Check sheet for the modelled part. Datum: model origin and axes. Units: mm. A direction names the side the tool comes from. Coordinates: 2 decimals unless noted, no trailing zeros. Loops run counter-clockwise (first coordinate to the right, second up) from the corner with the lowest first, then second, coordinate; pieces in that order, holes last.
```python
from build123d import *

# Parameters (mm, degrees)
F2_R     = 1.2
F3_DEPTH = 4.5
F4_R     = 0.75
F5_DEPTH = 7
F6_R     = 0.75
F7_DEPTH = 25
F9_DEPTH = 25


with BuildPart() as f1:
    # F0 (on Front) → F1 (revolve)
    with BuildSketch(Plane.XZ):
        with BuildLine():
            ThreePointArc((-16.2961422592, -2.25), (-18.5461422592, 0), (-16.2961422592, 2.25))
            Line((-16.2961422592, 2.25), (-19.7961422592, 2.25))
            Line((-19.7961422592, 2.25), (-19.7961422592, -2.25))
            Line((-19.7961422592, -2.25), (-16.2961422592, -2.25))
        make_face()
        with BuildLine():
            Line((-16.2961422592, 1.75), (-16.2961422592, 2.25))
            ThreePointArc((-16.2961422592, 2.25), (-18.5461422592, 0), (-16.2961422592, -2.25))
            Line((-16.2961422592, -2.25), (-16.2961422592, -1.75))
            ThreePointArc((-16.2961422592, -1.75), (-18.0461422592, 0), (-16.2961422592, 1.75))
        make_face()
    revolve(axis=Axis((-4.3961422592, 0, -0.5702087656), (0, 0, -1)))

    # F2 (on face) → F3 (join)
    with BuildSketch(Plane.XY.offset(2.25)):
        with BuildLine():
            ThreePointArc((-18.1132848188, -7), (-19.7961422592, 0), (-18.1132848188, 7))
            Line((-18.1132848188, 7), (-28.8961422592, 7))
            Line((-28.8961422592, 7), (-28.8961422592, -7))
            Line((-28.8961422592, -7), (-18.1132848188, -7))
        make_face()
        with Locations((-24.3961422592, 0)):
            Circle(F2_R, mode=Mode.SUBTRACT)
        with BuildLine():
            Line((16.3026824594, 4.5), (10.3317224876, 4.5))
            ThreePointArc((10.3317224876, 4.5), (10.8348970536, 2.2749596589), (11.0038577408, 0))
            ThreePointArc((11.0038577408, 0), (10.8348970536, -2.2749596589), (10.3317224876, -4.5))
            Line((10.3317224876, -4.5), (16.3026824594, -4.5))
            Line((16.3026824594, -4.5), (16.3026824594, 4.5))
        make_face()
    extrude(amount=-F3_DEPTH)

    # F4 (on face) → F5 (cut)
    with BuildSketch(Plane(origin=(0, 7, 0), x_dir=(-1, 0, 0), z_dir=(0, 1, 0))):
        with Locations((24.3961422592, 0)):
            Circle(F4_R)
    extrude(amount=-F5_DEPTH, mode=Mode.SUBTRACT)

    # F6 (on face) → F7 (cut)
    with BuildSketch(Plane(origin=(0, 4.5, 0), x_dir=(-1, 0, 0), z_dir=(0, 1, 0))):
        with Locations((-13.5026824594, 0)):
            Circle(F6_R)
    extrude(amount=-F7_DEPTH, mode=Mode.SUBTRACT)

    # F8 (on face) → F9 (cut)
    with BuildSketch(Plane.XY.offset(2.25)):
        with BuildLine():
            ThreePointArc((7.5038577408, 0), (7.50007322, 0.3000954384), (7.4887220648, 0.6))
            Line((7.4887220648, 0.6), (5.0247731139, 0.6))
            Line((5.0247731139, 0.6), (5.0247731139, -0.6))
            Line((5.0247731139, -0.6), (7.4887220648, -0.6))
            ThreePointArc((7.4887220648, -0.6), (7.50007322, -0.3000954384), (7.5038577408, 0))
        make_face()
        with BuildLine():
            Line((16.3026824594, -0.6), (16.3026824594, 0.6))
            Line((16.3026824594, 0.6), (7.4887220648, 0.6))
            ThreePointArc((7.4887220648, 0.6), (7.50007322, 0.3000954384), (7.5038577408, 0))
            ThreePointArc((7.5038577408, 0), (7.50007322, -0.3000954384), (7.4887220648, -0.6))
            Line((7.4887220648, -0.6), (16.3026824594, -0.6))
        make_face()
    extrude(amount=-F9_DEPTH, mode=Mode.SUBTRACT)


solid = f1.part
```
1) Mould release check, pull along Z, two halves, no side actions. Record for faces 4 (the cylindrical face through (14.252, 2.577, 0.033)), 5 (the cylindrical face through (-3.3, 15.36, -0.03)), 6 (the flat face through (-16.4, -1.1, -2.25)): +Z half, -Z half, draft (parallel to the pull), parting line (faces both ways), or undercut.
Answer sheet:
face 4: undercut
face 5: draft
face 6: -Z half
2) Section check A-A on z = 0. Enter the section's corners in (x, y).
Answer sheet:
outline: (-28.9, -7) - (-18.11, -7) arc R15.4 ccw to (10.33, -4.5) - (12.75, -4.5) - (12.75, -0.6) - (9.24, -0.6) arc R13.65 cw (long way) to (9.24, 0.6) - (12.75, 0.6) - (12.75, 4.5) - (10.33, 4.5) arc R15.4 ccw to (-18.11, 7) - (-23.65, 7) - (-23.65, 0.94) arc R1.2 cw (long way) to (-25.15, 0.94) - (-25.15, 7) - (-28.9, 7) - close; (14.25, -4.5) - (16.3, -4.5) - (16.3, -0.6) - (14.25, -0.6) - close; (14.25, 0.6) - (16.3, 0.6) - (16.3, 4.5) - (14.25, 4.5) - close
3) Scan lines: line 1 (Y direction, x = 13.5, z = 1.1); line 2 (X direction, y = -4, z = -0.9); line 3 (X direction, y = 5.5, z = 0.1). Record each from-to range of solid material in increasing order.
Answer sheet:
line 1: y = -4.5 to -0.6, 0.6 to 4.5
line 2: x = -28.9 to -17.19, 8.39 to 16.3
line 3: x = -28.9 to -25.14, -23.65 to -16.89, 8.09 to 9.99
4) Set-up check for faces 1 (the flat face through (13, 4.5, 1)), 2 (the flat face through (12, 0.6, 0)), 3 (the flat face through (-23, 7, 0)): record each of +Z, -Z, +X, -X, +Y, -Y from which the full face is reachable in a straight line by a thin tool's end or side.
Answer sheet:
face 1: +Z, -Z, +X, +Y
face 2: +Z, -Z, +X
face 3: +Z, -Z, -X, +Y
5) Depth check by flat-ended pin: pin 1 (14.5 mm diameter, centred on x = -4.4, y = 0, fed in from +Z); pin 2 (1.7 mm diameter, centred on x = 13.5, z = 0, fed in from -Y); pin 3 (1.7 mm diameter, centred on x = -24.4, z = 0, fed in from +Y); pin 4 (1 mm diameter, centred on x = -11, z = 0.5, fed in from -Y). Enter the tip coordinate at first touch or a pass-through.
Answer sheet:
pin 1: passes through
pin 2: stops at y = -4.5
pin 3: stops at y = 7
pin 4: stops at y = -14.14
